Input: dimensioned drawing with shaded views. Units: mm. Origin: part minimum x, y, z. Round coordinates to 2 decimals unless told otherwise and drop trailing zeros. Order: outer loops, then holes, each group sorted by start corner. A loop starts at its lowest first (then second) coordinate and runs counter-clockwise, first axis right, second up.
Item 1: Cut plane C-C on z = 57.5. Output: boundary loops of the cut face in (x, y) (1 decimal), then the cut area to 3 significant figures.
Item 2: First-contact query: pin 1 (1 mm diameter, centred on x = 53.5, y = 9, fed in from +Z); pin 2 (4 mm diameter, centred on y = 9.5, z = 44.5, fed in from -X); pin 3 (12 mm diameter, centred on x = 93.5, y = 3.5, fed in from +Z). Flat tips, straight axial feed; report the tip coordinate or a pass-through.
Item 3: Cut plane A-A on x = 101. Output: boundary loops of the cut face in (y, z).
Item 4: Mould query, pull axis Z, two halves, no side actions, for the marked faces 1, 2 and 3. Classes: released by +Z, released by -Z, zero draft, split by the parting line, or undercut.
Item 5: Cut plane B-B on z = 22. Output: boundary loops of the cut face in (x, y).
Item 6: Cut plane D-D on y = 5.25. Output: boundary loops of the cut face in (x, z) (1 decimal).
Item 7: Line query: L1, parallel to Z at x = 100, y = 23.5 (1 decimal); L2, parallel to Z at x = 103.5, y = 16.75 (1 decimal); L3, parallel to X at y = 9, z = 51.5 (1 decimal). Output: solid intervals per line, ascending.
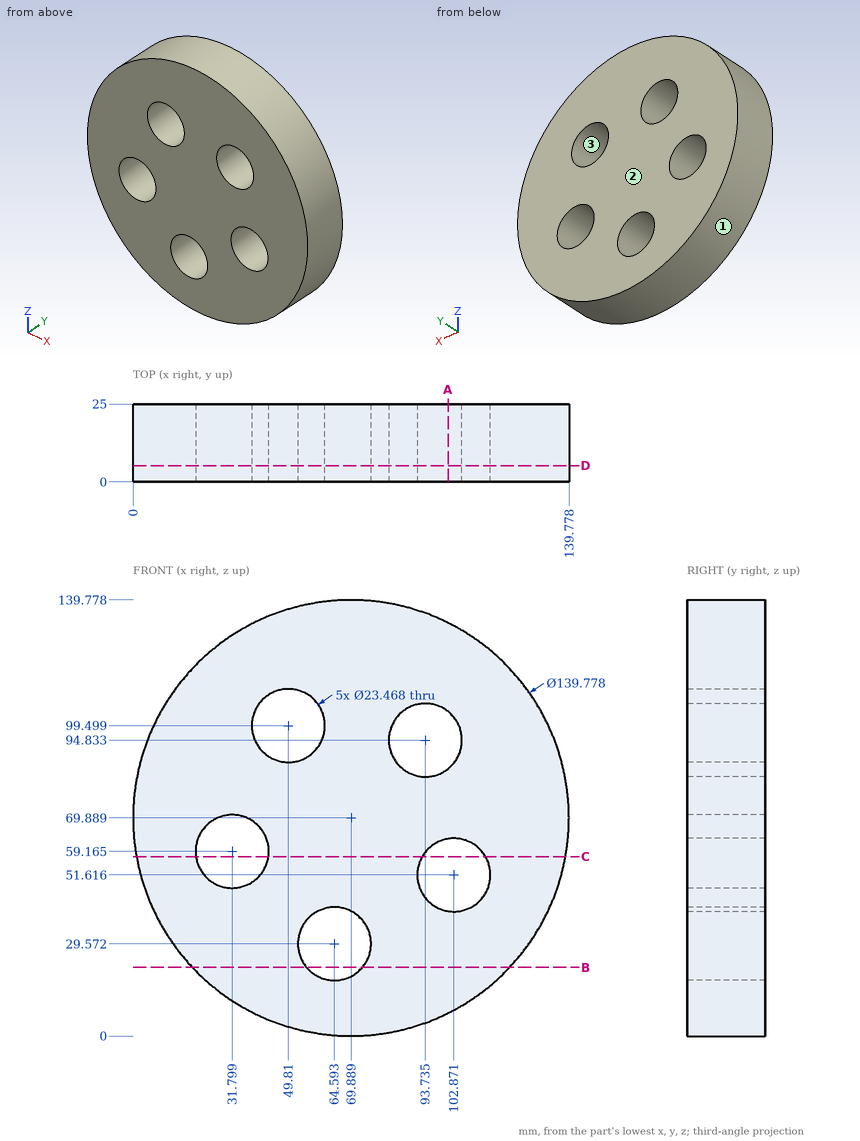
From the geometry:
1. outline: (1.1, 0) - (20.2, 0) - (20.2, 25) - (1.1, 25) - close; (43.4, 0) - (92.7, 0) - (92.7, 25) - (43.4, 25) - close; (113, 0) - (138.7, 0) - (138.7, 25) - (113, 25) - close
1. area: 2,350 mm2
2. pin 1: stops at z = 137.95
2. pin 2: stops at x = 4.03
2. pin 3: stops at z = 137.52
3. outline: (0, 7.31) - (25, 7.31) - (25, 40.03) - (0, 40.03) - close; (0, 63.2) - (25, 63.2) - (25, 85.62) - (0, 85.62) - close; (0, 104.05) - (25, 104.05) - (25, 132.47) - (0, 132.47) - close
4. face 1: split by the parting line
4. face 2: zero draft
4. face 3: undercut
5. outline: (18.99, 0) - (55.63, 0) - (55.63, 25) - (18.99, 25) - close; (73.56, 0) - (120.79, 0) - (120.79, 25) - (73.56, 25) - close
6. outline: circle Ø139.8 at (69.9, 69.9); hole circle Ø23.5 at (31.8, 59.2); hole circle Ø23.5 at (49.8, 99.5); hole circle Ø23.5 at (64.6, 29.6); hole circle Ø23.5 at (93.7, 94.8); hole circle Ø23.5 at (102.9, 51.6)
7. L1: z = 6.8 to 40.2, 63 to 84.9, 104.8 to 133
7. L2: z = 8.6 to 39.9, 63.3 to 88.3, 101.3 to 131.2
7. L3: x = 2.5 to 22.9, 40.7 to 91.1, 114.6 to 137.3
